Here's how the part is built. I have some questions about the finished solid (model axes, mm). A direction names the side the tool comes from. Coordinates: 2 decimals unless noted, no trailing zeros. Order: outer loops, then holes, each group sorted by start corner. A loop starts at its lowest first (then second) coordinate and runs counter-clockwise, first axis right, second up. Notation, with made-up numbers: (-15.75, 34.25) - (15.25, 34.25) arc R23 cw to (15.25, 63.25) - close; hole circle Ø3 at (-32.5, -38). An arc over 180 degrees is marked (long way). Answer in a Markdown table with one row per item. Add a question column.
Item 1: I want a section at A-A (y = -30). Please give me the cut outline in (x, z), plus the area to 3 significant figures.
Item 2: I want a section at B-B (x = 0). Please give me the cut outline in (y, z), plus the area to 3 significant figures.
Item 3: I want a section at D-D (y = -27.5). Please give me the cut outline in (x, z).
Item 4: Thinking about a two-plate mould opening in X: for faces 1 (the cylindrical face through (15.354, -17.042, 4.324)), 2 (the cylindrical face through (0.275, -32.497, 17.53)), 3 (the flat face through (22.5, -27, 11)), 4 (the flat face through (18, -14, 18)), which applies, +X half, -X half, draft (parallel to the pull), parting line (faces both ways), or undercut?
Item 5: Will these pins go through, and if not, where does the flat tip stop? pin 1 Ø8 at (x, z) = (-2.5, 17.5) entering from +Y; pin 2 Ø4 at (x, y) = (-16, -16) entering from -Z; pin 3 Ø2 at (x, z) = (5, 11.5) entering from +Y.
Item 6: I want a section at C-C (z = 5). Please give me the cut outline in (x, y).
Item 7: If I drill on line 1 along Z through (x, y) = (-10, -31.75); line 2 along X through (y, z) = (-27.5, 12); line 3 along Y through (x, z) = (0, 8.75), over which ranges is the centre line in solid material (lowest first)? Write a range as from..to.
Item 8: On a 3-axis mill with a long thin cutter (end or side, diameter ignored), from which of +Z, -Z, +X, -X, +Y, -Y can I reach the whole of each face in a straight line? I mean faces 5 (the cylindrical face through (-19.646, -17.042, 4.324)), 6 (the flat face through (-17, -14, 18)). Say none if no direction works.
Autodesk Fusion 360 part; units mm, degrees
sketch "スケッチ1" plane through (0, 0, 0) normal (0, 1, 0) x (1, 0, 0)
  line L0 (-21, 0) -> (21, 0)
  line L1 (21, 0) -> (21, -72.5)
  line L2 (21, -72.5) -> (-21, -72.5)
  line L3 (-21, -72.5) -> (-21, 0)
  line L4 (6.5, -72.5) -> (-6.5, -72.5)
  line L5 (-6.5, -72.5) -> (-6.5, -96.5)
  line L6 (-6.5, -96.5) -> (6.5, -96.5)
  line L7 (6.5, -96.5) -> (6.5, -72.5)
  line L8 (-12.5, -160.5) -> (9, -160.5)
  line L9 (9, -160.5) -> (9, -96.5)
  line L10 (9, -96.5) -> (-12.5, -96.5)
  line L11 (-12.5, -96.5) -> (-12.5, -160.5)
  line L12 (-21, -67.5) -> (21, -67.5) construction
  circle A0 centre (-12, -67.5) radius 1.75
  circle A1 centre (12, -67.5) radius 1.75
  line L13 (0, -1.75) -> (0, -22.5)
  circle A2 centre (0, -155.5) radius 2
  dimension "d1" = 42
  dimension "d2" = 5
  dimension "d3" = 3.5
  dimension "d4" = 3.5
  dimension "d5" = 24
  dimension "d6" = 72.5
  dimension "d7" = 13
  dimension "d8" = 2.5
  dimension "d9" = 6
  dimension "d10" = 24
  dimension "d11" = 64
  dimension "d12" = 4
  dimension "d13" = 5
extrude "押し出し1" add sketch "スケッチ1" against normal blind 2 makes body 1
sketch "スケッチ2" plane through (0, 0, 0) normal (0, 1, 0) x (-1, 0, 0)
  circle A0 centre (12, 67.5) radius 1.75
  circle A1 centre (-12, 67.5) radius 1.75
  circle A2 centre (0, 155.5) radius 2
  line L0 (6.5, 72.5) -> (6.5, 96.5)
  line L1 (6.5, 96.5) -> (12.5, 96.5)
  line L2 (12.5, 96.5) -> (12.5, 160.5)
  line L3 (12.5, 160.5) -> (-9, 160.5)
  line L4 (-9, 160.5) -> (-9, 96.5)
  line L5 (-9, 96.5) -> (-6.5, 96.5)
  line L6 (-6.5, 96.5) -> (-6.5, 72.5)
  line L7 (-6.5, 72.5) -> (-21, 72.5)
  line L8 (-21, 72.5) -> (-21, 0)
  line L9 (-21, 0) -> (21, 0)
  line L10 (21, 0) -> (21, 72.5)
  line L11 (21, 72.5) -> (6.5, 72.5)
  line L12 (-21, 0) -> (-22.5, 0)
  line L13 (-22.5, 0) -> (-22.5, 74)
  line L14 (-22.5, 74) -> (-8, 74)
  line L15 (-8, 74) -> (-8, 95)
  line L16 (-8, 95) -> (-10.5, 95)
  line L17 (-10.5, 95) -> (-10.5, 160.5)
  line L18 (-10.5, 160.5) -> (-9, 160.5)
  line L19 (12.5, 160.5) -> (14, 160.5)
  line L20 (14, 160.5) -> (14, 95)
  line L21 (14, 95) -> (8, 95)
  line L22 (8, 95) -> (8, 74)
  line L23 (8, 74) -> (22.5, 74)
  line L24 (22.5, 74) -> (22.5, 0)
  line L25 (22.5, 0) -> (21, 0)
  dimension "d16" = 1.5
  dimension "d17" = 1.5
  dimension "d18" = 1.5
  dimension "d19" = 1.5
  dimension "d20" = 1.5
  dimension "d22" = 1.5
  dimension "d23" = 1.5
  dimension "d24" = 1.5
  dimension "d25" = 1.5
  dimension "d26" = 1.5
extrude "押し出し2" add sketch "スケッチ2" against normal blind 15 contours L0 L1 L2 L10 L11 L19 L20 L21 L22 L23 L24 L25 | L4 L5 L6 L7 L8 L12 L13 L14 L15 L16 L17 L18 bodies 1
sketch "スケッチ3" plane through (0, -2, 0) normal (0, -1, 0) x (1, 0, 0)
  circle A0 centre (-12, 67.5) radius 1.75
  circle A1 centre (12, 67.5) radius 1.75
  circle A2 centre (0, 155.5) radius 2
  line L0 (-6.5, 96.5) -> (-6.5, 72.5)
  line L1 (-6.5, 72.5) -> (-21, 72.5)
  line L2 (-21, 72.5) -> (-21, 0)
  line L3 (-21, 0) -> (21, 0)
  line L4 (21, 0) -> (21, 72.5)
  line L5 (21, 72.5) -> (6.5, 72.5)
  line L6 (6.5, 72.5) -> (6.5, 96.5)
  line L7 (6.5, 96.5) -> (9, 96.5)
  line L8 (9, 96.5) -> (9, 160.5)
  line L9 (9, 160.5) -> (-12.5, 160.5)
  line L10 (-12.5, 160.5) -> (-12.5, 96.5)
  line L11 (-12.5, 96.5) -> (-6.5, 96.5)
  line L12 (-21, 0) -> (21, 0)
  line L13 (21, 0) -> (21, 10)
  line L14 (21, 10) -> (-21, 10)
  line L15 (-21, 10) -> (-21, 0)
  line L16 (-21, 12.6) -> (21, 12.6)
  line L17 (21, 12.6) -> (21, 22.6)
  line L18 (21, 22.6) -> (-21, 22.6)
  line L19 (-21, 22.6) -> (-21, 12.6)
  dimension "d29" = 10
  dimension "d30" = 10
  dimension "d31" = 2.6
extrude "押し出し3" add sketch "スケッチ3" along normal up to surface (13 mm away) contours L2 L4 L16 L17 L18 L19 | L2 L3 L4 L12 L13 L14 L15 bodies 1
sketch "スケッチ4" plane through (0, 0, 0) normal (0, 0, -1) x (1, 0, 0)
  line L0 (-22.5, 0) -> (22.5, 0)
  line L1 (22.5, 0) -> (22.5, 15)
  line L2 (22.5, 15) -> (-22.5, 15)
  line L3 (-22.5, 15) -> (-22.5, 0)
  arc A0 (-12.5, 15) -> (12.5, 15) centre (0, 15) ccw
  dimension "d34" = 25
extrude "押し出し4" cut sketch "スケッチ4" against normal up to surface (22.6 mm away) contours L2 A0 bodies 1
sketch "スケッチ10" plane through (0, -2, 0) normal (0, -1, 0) x (1, 0, 0)
  circle A0 centre (12, 67.5) radius 1.75
  circle A1 centre (0, 155.5) radius 2
  circle A2 centre (-12, 67.5) radius 1.75
  line L0 (-21, 22.6) -> (21, 22.6)
  line L1 (21, 22.6) -> (21, 72.5)
  line L2 (21, 72.5) -> (6.5, 72.5)
  line L3 (6.5, 72.5) -> (6.5, 96.5)
  line L4 (6.5, 96.5) -> (9, 96.5)
  line L5 (9, 96.5) -> (9, 160.5)
  line L6 (9, 160.5) -> (-12.5, 160.5)
  line L7 (-12.5, 160.5) -> (-12.5, 96.5)
  line L8 (-12.5, 96.5) -> (-6.5, 96.5)
  line L9 (-6.5, 96.5) -> (-6.5, 72.5)
  line L10 (-6.5, 72.5) -> (-21, 72.5)
  line L11 (-21, 72.5) -> (-21, 22.6)
  circle A3 centre (0, 155.5) radius 4
  dimension "d48" = 8
extrude "押し出し9" add sketch "スケッチ10" along normal blind 6 contours A3 bodies 1
sketch "スケッチ9" plane through (0, -2, 0) normal (0, -1, 0) x (1, 0, 0)
  circle A0 centre (12, 67.5) radius 1.75
  circle A1 centre (-12, 67.5) radius 1.75
  line L0 (-21, 22.6) -> (21, 22.6)
  line L1 (21, 22.6) -> (21, 72.5)
  line L2 (21, 72.5) -> (6.5, 72.5)
  line L3 (6.5, 72.5) -> (6.5, 96.5)
  line L4 (6.5, 96.5) -> (9, 96.5)
  line L5 (9, 96.5) -> (9, 160.5)
  line L6 (9, 160.5) -> (-12.5, 160.5)
  line L7 (-12.5, 160.5) -> (-12.5, 96.5)
  line L8 (-12.5, 96.5) -> (-6.5, 96.5)
  line L9 (-6.5, 96.5) -> (-6.5, 72.5)
  line L10 (-6.5, 72.5) -> (-21, 72.5)
  line L11 (-21, 72.5) -> (-21, 22.6)
  line L12 (-21, 72.5) -> (21, 72.5)
  line L13 (21, 72.5) -> (21, 62.5)
  line L14 (21, 62.5) -> (-21, 62.5)
  line L15 (-21, 62.5) -> (-21, 72.5)
  circle A2 centre (0, 155.5) radius 4
  dimension "d45" = 10
extrude "押し出し8" add sketch "スケッチ9" along normal blind 1 contours L1 L2 L10 L11 L12 L13 L14 L15 bodies 1
ref_plane "作業平面1" through (0, -20, 80.25) normal (0, -1, 0) x (0, 0, -1)
sketch "スケッチ6" plane through (0, -20, 0) normal (0, -1, 0) x (-1, 0, 0)
  line L0 (-22.5, 0) -> (22.5, 0)
  line L1 (22.5, 0) -> (22.5, -22.6)
  line L2 (22.5, -22.6) -> (-22.5, -22.6)
  line L3 (-22.5, -22.6) -> (-22.5, 0)
  line L4 (-22.5, 0) -> (-22.5, -74)
  line L5 (-12.5, -22.6) -> (-21, -22.6)
  line L6 (-12.5, 0) -> (-22.5, 0)
  line L7 (22.5, -74) -> (22.5, 0)
extrude "押し出し5" add sketch "スケッチ6" along normal blind 15 separate body makes body 2
sketch "スケッチ7" plane through (0, 0, 0) normal (0, 0, -1) x (1, 0, 0)
  line L0 (-22.5, 20) -> (22.5, 20)
  line L1 (22.5, 20) -> (22.5, 35)
  line L2 (22.5, 35) -> (-22.5, 35)
  line L3 (-22.5, 35) -> (-22.5, 20)
  arc A0 (12.5, 20) -> (-12.5, 20) centre (0, 20) ccw
  dimension "d40" = 25
extrude "押し出し6" cut sketch "スケッチ7" against normal up to surface (22.6 mm away) contours L0 A0 bodies 2
sketch "スケッチ8" plane through (0, -20, 0) normal (0, 1, 0) x (-1, 0, 0)
  line L0 (-12.5, 0) -> (-12.5, 22.6)
  line L1 (-12.5, 22.6) -> (-22.5, 22.6)
  line L2 (-22.5, 22.6) -> (-22.5, 0)
  line L3 (-22.5, 0) -> (-12.5, 0)
  line L4 (21, 12.6) -> (-21, 12.6)
  line L5 (-21, 12.6) -> (-21, 10)
  line L6 (-21, 10) -> (21, 10)
  line L7 (21, 10) -> (21, 12.6)
  point P0 (21, 12.6)
  point P1 (21, 10)
  point P2 (-21, 12.6)
extrude "押し出し7" cut sketch "スケッチ8" against normal blind 13 contours L0 L4 L5 L6 | L0 L4 L6 L7 bodies 2
sketch "スケッチ11" plane through (0, -15, 0) normal (0, -1, 0) x (1, 0, 0)
  line L0 (-12.5, 0) -> (-12.5, 10)
  line L1 (-12.5, 10) -> (-21, 10)
  line L2 (-21, 10) -> (-21, 12.6)
  line L3 (-21, 12.6) -> (-12.5, 12.6)
  line L4 (-12.5, 12.6) -> (-12.5, 22.6)
  line L5 (-12.5, 22.6) -> (-21, 22.6)
  line L6 (-21, 22.6) -> (-21, 72.5)
  line L7 (-21, 72.5) -> (-6.5, 72.5)
  line L8 (-6.5, 72.5) -> (-6.5, 96.5)
  line L9 (-6.5, 96.5) -> (-12.5, 96.5)
  line L10 (-12.5, 96.5) -> (-12.5, 160.5)
  line L11 (-12.5, 160.5) -> (-14, 160.5)
  line L12 (-14, 160.5) -> (-14, 95)
  line L13 (-14, 95) -> (-8, 95)
  line L14 (-8, 95) -> (-8, 74)
  line L15 (-8, 74) -> (-22.5, 74)
  line L16 (-22.5, 74) -> (-22.5, 0)
  line L17 (-22.5, 0) -> (-12.5, 0)
  line L18 (-17.5, 17.6) -> (17.5, 17.6) construction
  line L19 (17.5, 17.6) -> (17.5, 5) construction
  line L20 (17.5, 5) -> (-17.5, 5) construction
  line L21 (-17.5, 5) -> (-17.5, 17.6) construction
  line L22 (22.5, 0) -> (22.5, 74)
  circle A0 centre (-17.5, 17.6) radius 2.5
  circle A1 centre (17.5, 17.6) radius 2.5
  circle A2 centre (-17.5, 5) radius 2.5
  circle A3 centre (17.5, 5) radius 2.5
  dimension "d51" = 5
  dimension "d52" = 5
  dimension "d53" = 5
  dimension "d54" = 5
  dimension "d55" = 5
  dimension "d56" = 5
  dimension "d57" = 5
  dimension "d58" = 5
extrude "押し出し10" cut sketch "スケッチ11" against normal blind 10 contours A0 | A1 | A2 | A3 bodies 1
sketch "スケッチ12" plane through (0, -20, 0) normal (0, 1, 0) x (-1, 0, 0)
  line L0 (12.5, 12.6) -> (21, 12.6)
  line L1 (21, 12.6) -> (21, 10)
  line L2 (21, 10) -> (12.5, 10)
  line L3 (12.5, 10) -> (12.5, 0)
  line L4 (12.5, 0) -> (22.5, 0)
  line L5 (22.5, 0) -> (22.5, 22.6)
  line L6 (22.5, 22.6) -> (12.5, 22.6)
  line L7 (12.5, 22.6) -> (12.5, 12.6)
  circle A0 centre (17.5, 17.6) radius 2.5
  circle A1 centre (17.5, 17.6) radius 2.5
  circle A2 centre (17.5, 5) radius 2.5
  circle A3 centre (-17.5, 17.6) radius 2.5
  circle A4 centre (-17.5, 5) radius 2.5
  circle A5 centre (-17.5, 17.6) radius 2.25
  circle A6 centre (-17.5, 5) radius 2.25
  circle A7 centre (17.5, 17.6) radius 2.25
  circle A8 centre (17.5, 5) radius 2.25
  dimension "d63" = 4.5
  dimension "d64" = 4.5
  dimension "d65" = 4.5
  dimension "d66" = 4.5
extrude "押し出し12" add sketch "スケッチ12" along normal blind 6 contours A5 | A6 | A7 | A8 bodies 2
sketch "スケッチ14" plane through (0, 0, 0) normal (0, 1, 0) x (-1, 0, 0)
  circle A0 centre (0, 155.5) radius 2
  circle A1 centre (12, 67.5) radius 1.75
  circle A2 centre (-12, 67.5) radius 1.75
  line L0 (14, 160.5) -> (-10.5, 160.5)
  line L1 (-10.5, 160.5) -> (-10.5, 95)
  line L2 (-10.5, 95) -> (-8, 95)
  line L3 (-8, 95) -> (-8, 74)
  line L4 (-8, 74) -> (-22.5, 74)
  line L5 (-22.5, 74) -> (-22.5, 0)
  line L6 (-22.5, 0) -> (22.5, 0)
  line L7 (22.5, 0) -> (22.5, 74)
  line L8 (22.5, 74) -> (8, 74)
  line L9 (8, 74) -> (8, 95)
  line L10 (8, 95) -> (14, 95)
  line L11 (14, 95) -> (14, 160.5)
  line L12 (14, 149) -> (15.5, 149)
  line L13 (15.5, 149) -> (14, 150.5)
  line L14 (14, 126.5) -> (15.5, 126.5)
  line L15 (15.5, 126.5) -> (14, 125)
  line L16 (-10.5, 150.5) -> (-12, 149)
  line L17 (-12, 149) -> (-10.5, 149)
  line L18 (-10.5, 126.5) -> (-12, 126.5)
  line L19 (-12, 126.5) -> (-10.5, 125)
  dimension "d79" = 10
  dimension "d80" = 10
  dimension "d81" = 1.5
  dimension "d82" = 1.5
  dimension "d83" = 22.5
  dimension "d84" = 1.5
  dimension "d85" = 1.5
  dimension "d86" = 1.5
  dimension "d88" = 1.5
  dimension "d89" = 1.5
extrude "押し出し13" add sketch "スケッチ14" against normal up to surface (15 mm away) contours L11 L12 L13 | L1 L16 L17 | L11 L14 L15 | L1 L18 L19 bodies 1
hidden bodies 1
Values follow:
| question | item | result |
|---|---|---|
| 1 | outline | (-22.5, 0) - (-7.5, 0) - (-7.5, 10) - (-21, 10) - (-21, 12.6) - (-7.5, 12.6) - (-7.5, 22.6) - (-22.5, 22.6) - close; (7.5, 0) - (22.5, 0) - (22.5, 22.6) - (7.5, 22.6) - (7.5, 12.6) - (21, 12.6) - (21, 10) - (7.5, 10) - close |
| 1 | area | 608 mm^2 |
| 2 | outline | (-35, 0) - (-32.5, 0) - (-32.5, 10) - (-33, 10) - (-33, 12.6) - (-32.5, 12.6) - (-32.5, 22.6) - (-35, 22.6) - close |
| 2 | area | 55.2 mm^2 |
| 3 | outline | (-22.5, 0) - (-10, 0) - (-10, 10) - (-21, 10) - (-21, 12.6) - (-10, 12.6) - (-10, 22.6) - (-22.5, 22.6) - close; (10, 0) - (22.5, 0) - (22.5, 22.6) - (10, 22.6) - (10, 12.6) - (21, 12.6) - (21, 10) - (10, 10) - close |
| 4 | face 1 | undercut |
| 4 | face 2 | undercut |
| 4 | face 3 | +X half |
| 4 | face 4 | draft |
| 5 | pin 1 | stops at y = -30.68 |
| 5 | pin 2 | stops at z = 2.75 |
| 5 | pin 3 | stops at y = -33 |
| 6 | outline | (-22.5, -35) - (22.5, -35) - (22.5, -20) - (19.75, -20) - (19.75, -14) - (15.25, -14) - (15.25, -20) - (12.5, -20) arc R12.5 cw to (-12.5, -20) - (-15.25, -20) - (-15.25, -14) - (-19.75, -14) - (-19.75, -20) - (-22.5, -20) - close |
| 7 | line 1 | z = 0..10, 12.6..22.6 |
| 7 | line 2 | x = -22.5..-21, 21..22.5 |
| 7 | line 3 | y = -35..-32.5 |
| 8 | face 5 | +Y |
| 8 | face 6 | +Z, -Z, +X, -X, +Y |
